For this review, take the finished solid that the model builds, in its own axes (mm). Face numbers are marked on the shaded views. Round coordinates to 2 decimals unless told otherwise and drop trailing zeros. Order: outer loops, then holes, each group sorted by start corner. A loop starts at its lowest first (then second) coordinate and runs counter-clockwise, first axis right, second up.
```python
from build123d import *

# Parameters (mm, degrees)
SKETCH1_W           = 28.5
SKETCH1_H           = 15.2
BOSS_EXTRUDE1_DEPTH = 1
SKETCH5_R           = 0.75
BOSS_EXTRUDE4_DEPTH = 5


with BuildPart() as part:
    # Sketch1 → Boss-Extrude1 (new body)
    with BuildSketch(Plane(origin=(0, 0, 0), x_dir=(1, 0, 0), z_dir=(0, 1, 0))):
        with Locations((14.25, 7.6)):
            Rectangle(SKETCH1_W, SKETCH1_H)
    extrude(amount=BOSS_EXTRUDE1_DEPTH)

    # Sketch5 → Boss-Extrude4 (add)
    with BuildSketch(Plane(origin=(0, 1, 0), x_dir=(1, 0, 0), z_dir=(0, 1, 0))):
        with Locations(Location((27, 1.5, 0), (0, 0, 270))):
            Circle(SKETCH5_R)
        with Locations(Location((24.46, 1.5, 0), (0, 0, 270))):
            Circle(SKETCH5_R)
        with Locations(Location((24.46, 4.04, 0), (0, 0, 270))):
            Circle(SKETCH5_R)
        with Locations(Location((27, 4.04, 0), (0, 0, 270))):
            Circle(SKETCH5_R)
        with Locations(Location((24.46, 6.58, 0), (0, 0, 270))):
            Circle(SKETCH5_R)
        with Locations(Location((27, 6.58, 0), (0, 0, 270))):
            Circle(SKETCH5_R)
        with Locations(Location((24.46, 9.12, 0), (0, 0, 270))):
            Circle(SKETCH5_R)
        with Locations(Location((27, 9.12, 0), (0, 0, 270))):
            Circle(SKETCH5_R)
    extrude(amount=-BOSS_EXTRUDE4_DEPTH)


solid = part.part
```
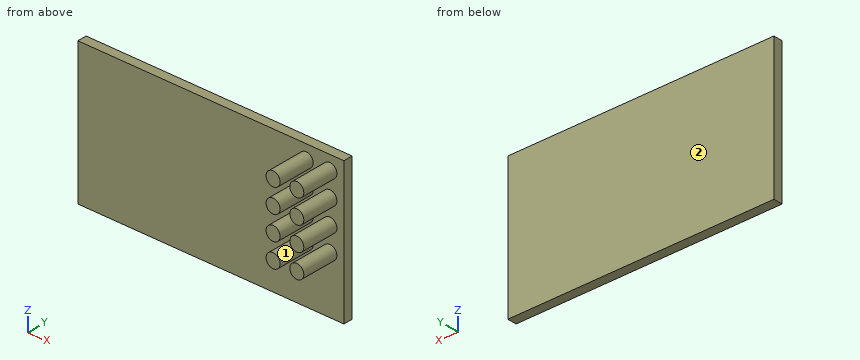
Q1. Take a section at D-D, the plane z = -11. State the section outline as (x, y) points, plus the area to 3 significant figures.
Q2. Take a section at B-B, the plane z = -6.58. State the section outline as (x, y) points.
Q3. Wall thickness on line 1 (X direction, y = -2.25, z = -4); line 2 (Y direction, x = 15, z = -8.25); line 3 (X direction, y = -1.4, z = -9.5): over which ranges is each line inside the solid? List them lowest first.
Q4. Clearance check with flat-ended pins moving along their axes: pin 1 (1.5 mm diameter, centred on y = 0.5, z = -8.5, fed in from -X); pin 2 (1 mm diameter, centred on y = -2.5, z = -5.5, fed in from +X); pin 3 (8 mm diameter, centred on x = 7.5, z = -5.5, fed in from -Y). State where each tip first meets the part, or that it passes through.
Q5. Take a section at C-C, the plane x = 24.46. State the section outline as (y, z) points, plus the area to 3 significant figures.
Q6. Mouldability with a two-part tool opening along Z and no side actions: class the marked faces 1 and 2 as +Z half, -Z half, draft (parallel to the pull), parting line (faces both ways), or undercut.
Q7. Take a section at A-A, the plane y = -1.7. State the section outline as (x, z) points.
Working result:
1. outline: (0, 0) - (28.5, 0) - (28.5, 1) - (0, 1) - close
1. area: 28.5 mm2
2. outline: (0, 0) - (23.71, 0) - (23.71, -4) - (25.21, -4) - (25.21, 0) - (26.25, 0) - (26.25, -4) - (27.75, -4) - (27.75, 0) - (28.5, 0) - (28.5, 1) - (0, 1) - close
3. line 1: x = 23.71 to 25.21, 26.25 to 27.75
3. line 2: y = 0 to 1
3. line 3: x = 23.81 to 25.11, 26.35 to 27.65
4. pin 1: stops at x = 0
4. pin 2: stops at x = 27.48
4. pin 3: stops at y = 0
5. outline: (-4, -9.87) - (0, -9.87) - (0, -15.2) - (1, -15.2) - (1, 0) - (0, 0) - (0, -0.75) - (-4, -0.75) - (-4, -2.25) - (0, -2.25) - (0, -3.29) - (-4, -3.29) - (-4, -4.79) - (0, -4.79) - (0, -5.83) - (-4, -5.83) - (-4, -7.33) - (0, -7.33) - (0, -8.37) - (-4, -8.37) - close
5. area: 39.2 mm2
6. face 1: undercut
6. face 2: draft
7. outline: circle Ø1.5 at (24.46, -9.12); circle Ø1.5 at (24.46, -6.58); circle Ø1.5 at (24.46, -4.04); circle Ø1.5 at (24.46, -1.5); circle Ø1.5 at (27, -9.12); circle Ø1.5 at (27, -6.58); circle Ø1.5 at (27, -4.04); circle Ø1.5 at (27, -1.5)
